Source: CAD feature listing. Evaluate the final solid. Frame: model axes, mm. A direction names the side the tool comes from. Round coordinates to 2 decimals unless told otherwise and drop trailing zeros. Order: outer loops, then holes, each group sorted by start corner. A loop starts at its lowest first (then second) coordinate and runs counter-clockwise, first axis right, second up. Notation, with made-up numbers: (26, 75) - (43, 75) arc R16 ccw to (43, 90) - close; hole circle Ø10 at (-37.5, 78). An arc over 180 degrees is marked (long way). Put each result on its own line as item: value. Start each with the question number.
1) Section D-D on z = 84.5. Output: boundary loops of the cut face in (x, y).
2) Access query for faces 4 (the face through (-1.575, -101.488, 245.07)), 5 (the face through (0, -102, 0)). Directions: +Z, -Z, +X, -X, +Y, -Y. A direction counts if a zero-diameter tool reaches every point of the face in a straight line with its end or side. Return the directions, or none.
3) Contact query for flat-ended pins moving along their axis: P1, Ø8, axis at x = -43, z = 200.5, coming from the -Y side; P2, Ø1, axis at x = 65, z = 41.5, coming from the -Y side; P3, Ø1, axis at x = -3, z = 218.5, coming from the -Y side. Output: stop coordinate, or through.
4) Section A-A on y = -70.5. Output: boundary loops of the cut face in (x, z), then the cut area to 3 significant figures.
5) Section C-C on y = -87. Output: boundary loops of the cut face in (x, z).
6) Line query: probe 1 along X at (y, z) = (-86, 68.5); probe 2 along X at (y, z) = (-90.5, 218); probe 3 along Y at (x, z) = (-16, 203.5). Output: solid intervals per line, ascending. Write a range as [from, to].
7) Mould query, pull axis X, two halves, no side actions, for faces 1 (the face through (6, -100, 250)), 2 (the face through (-1.598, -102.988, 118.32)), 3 (the face through (1.552, -99.988, 123.25)). Classes: +X half, -X half, draft (parallel to the pull), parting line (faces both ways), or undercut.
8) Section B-B on x = 79. Output: boundary loops of the cut face in (y, z).
```python
from build123d import *

# Parameters (mm, degrees)
F1_DEPTH = 250
F2_R     = 103
F2_R_2   = 101.5
F3_DEPTH = 10


with BuildPart() as f1:
    # F0 (on Top) → F1 (new body)
    with BuildSketch(Plane.XY):
        with BuildLine():
            Line((-89.493436, -44.619781), (-92.178239, -45.958375))
            ThreePointArc((-92.178239, -45.958375), (0, -103), (92.178239, -45.958375))
            Line((92.178239, -45.958375), (89.493436, -44.619781))
            ThreePointArc((89.493436, -44.619781), (0, -100), (-89.493436, -44.619781))
        make_face()
    extrude(amount=F1_DEPTH)

    # F2 (on face) → F3 (cut)
    with BuildSketch(Plane.XY.offset(250)):
        Circle(F2_R)
        Circle(F2_R_2, mode=Mode.SUBTRACT)
    extrude(amount=-F3_DEPTH, mode=Mode.SUBTRACT)


solid = f1.part
```
Answer sheet:
1. outline: (-92.18, -45.96) arc R103 ccw to (92.18, -45.96) - (89.49, -44.62) arc R100 cw to (-89.49, -44.62) - close
2. face 4: +Z, -Y
2. face 5: -Z, +X, -X, +Y, -Y
3. P1: y = -95.33
3. P2: y = -80.3
3. P3: y = -102.97
4. outline: (-75.09, 0) - (-70.92, 0) - (-70.92, 250) - (-73.02, 250) - (-73.02, 240) - (-75.09, 240) - close; (70.92, 0) - (75.09, 0) - (75.09, 240) - (73.02, 240) - (73.02, 250) - (70.92, 250) - close
4. area: 2,040 mm^2
5. outline: (-55.14, 0) - (-49.31, 0) - (-49.31, 250) - (-52.28, 250) - (-52.28, 240) - (-55.14, 240) - close; (49.31, 0) - (55.14, 0) - (55.14, 240) - (52.28, 240) - (52.28, 250) - (49.31, 250) - close
6. probe 1: [-56.68, -51.03], [51.03, 56.68]
6. probe 2: [-49.18, -42.54], [42.54, 49.18]
6. probe 3: [-101.75, -98.71]
7. face 1: draft
7. face 2: parting line
7. face 3: undercut
8. outline: (-66.09, 0) - (-61.31, 0) - (-61.31, 250) - (-63.73, 250) - (-63.73, 240) - (-66.09, 240) - close
